Input: part model. Units: mm. Frame: model coordinates. Face numbers are marked on the shaded views. Give positions to 0.01 mm unless a question says otherwise; leave off trailing zeros. Loops run counter-clockwise (first coordinate to the right, second up) from the corner with the lowest first, then second, coordinate; pieces in that order, holes last. Notation, with made-up numbers: M 70,4.5 L 77,4.5 A17 ccw 77,20.5 Z; hole C 54,81 d4. An arc over 180 degrees is marked long. Use a Markdown table: item, result. Add a question column.
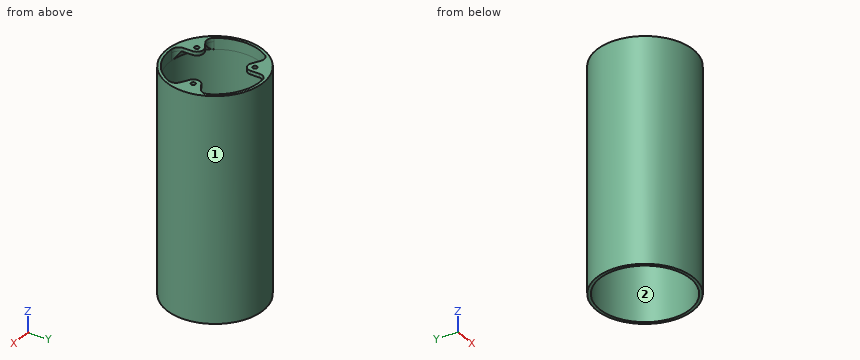
from build123d import *

# Parameters (mm, degrees)
SKETCH1_R           = 32.5
SKETCH1_R_2         = 30.5
BOSS_EXTRUDE1_DEPTH = 150
BOSS_EXTRUDE2_START = -2.5
SKETCH2_R           = 1.55
BOSS_EXTRUDE2_DEPTH = 2.5
FILLET1_R           = 5
CHAMFER1_START      = 142.49999956
CHAMFER1_DEPTH      = 5.00000044
CHAMFER1_START_2    = 142.499980406
CHAMFER1_3_DEPTH    = 5.000019594


with BuildPart() as part:
    # Sketch1 → Boss-Extrude1 (new body)
    with BuildSketch(Plane.XY):
        Circle(SKETCH1_R)
        Circle(SKETCH1_R_2, mode=Mode.SUBTRACT)
    extrude(amount=BOSS_EXTRUDE1_DEPTH)

    # Sketch2 → Boss-Extrude2 (add)
    # profile 1 of 3: a face of its own
    with BuildSketch(Plane.XY.offset(150).offset(BOSS_EXTRUDE2_START)):
        with BuildLine():
            Line((20.225, -3.940415587), (29.118585526, -9.075129585))
            ThreePointArc((29.118585526, -9.075129585), (30.152668692, -4.58983341), (30.5, 0))
            ThreePointArc((30.5, 0), (30.152668692, 4.58983341), (29.118585526, 9.075129585))
            Line((29.118585526, 9.075129585), (20.225, 3.940415587))
            ThreePointArc((20.225, 3.940415587), (17.95, 0), (20.225, -3.940415587))
        make_face()
        with Locations((22.5, 0)):
            Circle(SKETCH2_R, mode=Mode.SUBTRACT)
    # profile 2 of 3: a face of its own
    with BuildSketch(Plane.XY.offset(150).offset(BOSS_EXTRUDE2_START)):
        with BuildLine():
            ThreePointArc((-6.7, 29.75499958), (-15.25, 26.413774815), (-22.418585526, 20.679869995))
            Line((-22.418585526, 20.679869995), (-13.525, 15.545155998))
            ThreePointArc((-13.525, 15.545155998), (-8.975, 15.545155998), (-6.7, 19.485571585))
            Line((-6.7, 19.485571585), (-6.7, 29.75499958))
        make_face()
        with Locations((-11.25, 19.485571585)):
            Circle(SKETCH2_R, mode=Mode.SUBTRACT)
    # profile 3 of 3: a face of its own
    with BuildSketch(Plane.XY.offset(150).offset(BOSS_EXTRUDE2_START)):
        with BuildLine():
            ThreePointArc((-22.418585526, -20.679869995), (-15.25, -26.413774815), (-6.7, -29.75499958))
            Line((-6.7, -29.75499958), (-6.7, -19.485571585))
            ThreePointArc((-6.7, -19.485571585), (-8.975, -15.545155998), (-13.525, -15.545155998))
            Line((-13.525, -15.545155998), (-22.418585526, -20.679869995))
        make_face()
        with Locations((-11.25, -19.485571585)):
            Circle(SKETCH2_R, mode=Mode.SUBTRACT)
    extrude(amount=BOSS_EXTRUDE2_DEPTH)

    # Fillet1
    fillet1_edges = [part.edges().sort_by_distance(p)[0] for p in [
        (29.118585526, 9.075129585, 148.75),
        (29.118585526, -9.075129585, 148.75),
        (-22.418585526, 20.679869995, 148.75),
        (-6.7, 29.75499958, 148.75),
        (-6.7, -29.75499958, 148.75),
        (-22.418585526, -20.679869995, 148.75),
    ]]
    fillet(fillet1_edges, radius=FILLET1_R)

    # Chamfer1: read off the stored shape, not the designer's step
    # Chamfer1 outline → Chamfer1 (add)
    with BuildSketch(Plane.XY.offset(CHAMFER1_START)):
        with BuildLine():
            ThreePointArc((27.37167884, -13.455155052), (30.5, 0), (27.37167884, 13.455155052))
            ThreePointArc((27.37167884, 13.455155052), (15.25, 26.413774815), (-2.033333333, 30.432146746))
            ThreePointArc((-2.033333333, 30.432146746), (-15.25, 26.413774816), (-25.338345507, 16.976991694))
            ThreePointArc((-25.338345507, 16.976991694), (-30.5, 0), (-25.338345507, -16.976991694))
            ThreePointArc((-25.338345507, -16.976991694), (-15.25, -26.413774816), (-2.033333333, -30.432146746))
            ThreePointArc((-2.033333333, -30.432146746), (15.25, -26.413774815), (27.37167884, -13.455155052))
        make_face()
    extrude(amount=CHAMFER1_DEPTH)

    # Chamfer1 2 outline → Chamfer1 2 (revolve, cut)
    with BuildSketch(Plane.XZ):
        Polygon((0, 142.499980406), (30.500011313, 142.499980406), (27.613248654, 147.5), (0, 147.5), align=None)
    revolve(axis=Axis((0, 0, 0), (0, 0, 1)), mode=Mode.SUBTRACT)

    # Chamfer1 3 outline → Chamfer1 3 (cut)
    with BuildSketch(Plane.XY.offset(CHAMFER1_START_2)):
        with BuildLine():
            ThreePointArc((-2.033333333, 30.432146746), (-4.834338384, 29.33889892), (-6.501863856, 26.836863968))
            ThreePointArc((-6.501863856, 26.836863968), (13.806624327, 23.913774815), (26.492337882, 7.787652712))
            ThreePointArc((26.492337882, 7.787652712), (27.825400976, 10.482789609), (27.37167884, 13.455155052))
            ThreePointArc((27.37167884, 13.455155052), (15.25, 26.413774815), (-2.033333333, 30.432146746))
        make_face()
        with BuildLine():
            ThreePointArc((26.492337882, -7.787652712), (13.806624327, -23.913774815), (-6.501863856, -26.836863968))
            ThreePointArc((-6.501863856, -26.836863968), (-4.834338384, -29.33889892), (-2.033333333, -30.432146746))
            ThreePointArc((-2.033333333, -30.432146746), (15.25, -26.413774815), (27.37167884, -13.455155052))
            ThreePointArc((27.37167884, -13.455155052), (27.825400976, -10.482789609), (26.492337882, -7.787652712))
        make_face()
        with BuildLine():
            ThreePointArc((-25.338345507, 16.976991694), (-30.5, 0), (-25.338345507, -16.976991694))
            ThreePointArc((-25.338345507, -16.976991694), (-22.991062592, -18.856109312), (-19.990474026, -19.049211255))
            ThreePointArc((-19.990474026, -19.049211255), (-27.613248654, 0), (-19.990474026, 19.049211255))
            ThreePointArc((-19.990474026, 19.049211255), (-22.991062592, 18.856109311), (-25.338345507, 16.976991694))
        make_face()
    extrude(amount=CHAMFER1_3_DEPTH, mode=Mode.SUBTRACT)


solid = part.part
1) Pull-direction query (Y, two-part tool) for the marked faces 1 and 2; classes: pulls with the +Y half, pulls with the -Y half, needs draft (parallel to the pull), parting line crosses it, or undercut.
2) Contact query for flat-ended pins moving along their axis: P1, Ø6, axis at x = 2, z = 60, coming from the -Y side; P2, Ø1.5, axis at y = -17, z = 17, coming from the +X side; P3, Ø1.5, axis at x = -7.5, z = 37, coming from the +Y side; P4, Ø1.9, axis at x = -11.25, y = 19.49, coming from the +Z side. Output: stop coordinate, or through.
3) Ray query, line 1 (Y direction, x = -11.25, z = 149.45); line 2 (Y direction, x = 0, z = 107); line 3 (Y direction, x = -11, z = 148). Return the intervals inside material, ascending. Write a range as [from, to].
4) Section query D-D, the plane x = 22.5. State how many separate pieces and enclosed holes the cut face has, and give its area (3 significant figures).
5) Section query C-C, the plane x = -27. Return the cut outline in (y, z).
6) Section query B-B, the plane z = 67. Return the cut outline in (x, y).
Entries:
| question | item | result |
|---|---|---|
| 1 | face 1 | parting line crosses it |
| 1 | face 2 | undercut |
| 2 | P1 | stops at y = -32.5 |
| 2 | P2 | stops at x = 28.15 |
| 2 | P3 | stops at y = 31.79 |
| 2 | P4 | passes through |
| 3 | line 1 | y = [-30.49, -21.04], [-17.94, -14.94], [14.94, 17.94], [21.04, 30.49] |
| 3 | line 2 | y = [-32.5, -30.5], [30.5, 32.5] |
| 3 | line 3 | y = [-30.58, -21.02], [-17.96, -14.94], [14.94, 17.96], [21.02, 30.58] |
| 4 | separate pieces | 4 |
| 4 | enclosed holes | 0 |
| 4 | area | 877 mm² |
| 5 | outline | M -18.09,0 L -14.19,0 L -14.19,150 L -18.09,150 Z; M 14.19,0 L 18.09,0 L 18.09,150 L 14.19,150 Z |
| 6 | outline | C 0,0 d65; hole C 0,0 d61 |
